The listing builds one solid part. Answer for the finished solid, in the listing's coordinates (mm). A direction names the side the tool comes from. Coordinates: 2 decimals unless noted, no trailing zeros. Loops run counter-clockwise (first coordinate to the right, second up) from the corner with the lowest first, then second, coordinate; pieces in that order, holes last. Notation, with made-up numbers: (51.5, 83) -> (86.5, 83) arc R20 ccw to (86.5, 95) -> close; hole circle Ø11 at (79.5, 50). An arc over 180 degrees is marked (long way). Answer in a Markdown table with one row per item.
Autodesk Inventor part; units mm, degrees
ref_plane "YZ Plane" through (0, 0, 0) normal (1, 0, 0) x (0, 1, 0)
ref_plane "XZ Plane" through (0, 0, 0) normal (0, 1, 0) x (-1, 0, 0)
ref_plane "XY Plane" through (0, 0, 0) normal (0, 0, 1) x (1, 0, 0)
sketch "Sketch1" plane through (0, 0, 0) normal (1, 0, 0) x (0, 1, 0)
  line L0 (0, 0) -> (21.5, 0)
  line L1 (21.5, 0) -> (21.5, -6.35) construction
  line L2 (21.5, -27.85) -> (0, -27.85)
  line L3 (0, -27.85) -> (0, -6.35) construction
  line L4 (21.5, 0) -> (27.85, 0)
  line L5 (27.85, 0) -> (27.85, -34.2)
  line L6 (-6.35, -34.2) -> (-6.35, -6.35) construction
  line L7 (-6.35, 0) -> (0, 0)
  line L8 (27.85, -34.2) -> (-6.35, -34.2)
  line L9 (-6.35, 0) -> (-57.15, 0)
  line L10 (-57.15, 0) -> (-57.15, -82.55)
  line L11 (-6.35, -6.35) -> (-50.8, -6.35)
  line L12 (-50.8, -6.35) -> (-50.8, -76.2)
  line L13 (-6.35, -6.35) -> (-6.35, 0) construction
  line L14 (-57.15, -82.55) -> (-3.7197, -82.55)
  line L15 (-50.8, -76.2) -> (-6.35, -76.2)
  line L16 (-6.35, -76.2) -> (11.6105, -58.2395)
  line L17 (-3.7197, -82.55) -> (11.6105, -67.2197)
  line L18 (11.6105, -58.2395) -> (11.6105, -67.2197)
  line L19 (-6.35, -34.2) -> (-6.35, -76.2) construction
  line L20 (0, -6.35) -> (21.5, -6.35)
  line L21 (0, -6.35) -> (-6.35, -6.35)
  line L22 (0, -6.35) -> (0, 0) construction
  line L23 (21.5, -6.35) -> (21.5, -27.85)
  line L24 (0, -27.85) -> (-6.35, -34.2)
  dimension "d2" = 6.35
  dimension "d4" = 6.35
  dimension "d23" = 6.35
  dimension "d24" = 50.8
  dimension "d25" = 82.55
  dimension "d26" = 6.35
  dimension "d27" = 6.35
  dimension "d28" = 6.35
  dimension "d30" = 6.35
  dimension "d31" = 25.4
  dimension "d32" = 135
  dimension "d33" = 21.5
  dimension "d34" = 6.35
  dimension "d35" = 21.5
  dimension "d36" = 24.0395
extrude "Extrusion1" add sketch "Sketch1" along normal blind 6.35
equation "\"d35\" = d33"
properties part number "Main"
Item 1: A cutting plane is placed at B-B, the plane y = -31.5. Determine the outline of the cut face in (x, z).
Findings below:
| item | result |
|---|---|
| outline | (0, -82.55) -> (6.35, -82.55) -> (6.35, -76.2) -> (0, -76.2) -> close; (0, -6.35) -> (6.35, -6.35) -> (6.35, 0) -> (0, 0) -> close |
Item 2: A cutting plane is placed at D-D, the plane y = -2.5. Determine the outline of the cut face in (x, z).
Findings below:
| item | result |
|---|---|
| outline | (0, -81.33) -> (6.35, -81.33) -> (6.35, -72.35) -> (0, -72.35) -> close; (0, -34.2) -> (6.35, -34.2) -> (6.35, -30.35) -> (0, -30.35) -> close; (0, -6.35) -> (6.35, -6.35) -> (6.35, 0) -> (0, 0) -> close |
Item 3: Find the intervals of material crossed by probe 1 along Y at (x, z) = (5.25, -18.5); probe 2 along Z at (x, y) = (4.5, -18); probe 3 along Z at (x, y) = (4, 6), in increasing order.
Findings below:
| item | result |
|---|---|
| probe 1 | y = -57.15 to -50.8, 21.5 to 27.85 |
| probe 2 | z = -82.55 to -76.2, -6.35 to 0 |
| probe 3 | z = -72.83 to -63.85, -34.2 to -27.85, -6.35 to 0 |
Item 4: Determine the mould class of faces 4 (the face through (0, 1, -29)), 5 (the face through (3.13, 2.5, -67.35)), 6 (the face through (3, -14, 0)) for opening direction Z: +Z half, -Z half, draft (parallel to the pull), parting line (faces both ways), or undercut.
Findings below:
| item | result |
|---|---|
| face 4 | draft |
| face 5 | undercut |
| face 6 | +Z half |
Item 5: A tool of negligible diameter and unlimited length cuts with its end or side. For faces 1 (the face through (3, 11, -34.2)), 2 (the face through (3, 21.5, -17)), 3 (the face through (3, 11.61, -63)), from which of +Z, -Z, +X, -X, +Y, -Y can it reach the whole face along a straight path? Write none if from no direction.
Findings below:
| item | result |
|---|---|
| face 1 | +X, -X, +Y |
| face 2 | +X, -X |
| face 3 | -Z, +X, -X, +Y |
Item 6: A cutting plane is placed at C-C, the plane x = 2.25. Determine the outline of the cut face in (y, z), plus the area to 3 significant figures.
Findings below:
| item | result |
|---|---|
| outline | (-57.15, -82.55) -> (-3.72, -82.55) -> (11.61, -67.22) -> (11.61, -58.24) -> (-6.35, -76.2) -> (-50.8, -76.2) -> (-50.8, -6.35) -> (21.5, -6.35) -> (21.5, -27.85) -> (0, -27.85) -> (-6.35, -34.2) -> (27.85, -34.2) -> (27.85, 0) -> (-57.15, 0) -> close |
| area | 1,800 mm2 |
Item 7: Flat-ended cylindrical pins translate along their axes: pin 1 Ø3 at (x, z) = (3.5, -37) entering from +Y; pin 2 Ø1.5 at (x, y) = (1.5, -13) entering from +Z; pin 3 Ø6 at (y, z) = (-8, -71.5) entering from -X. Find the tip coordinate at first contact, or state that the pin passes through.
Findings below:
| item | result |
|---|---|
| pin 1 | stops at y = -50.8 |
| pin 2 | stops at z = 0 |
| pin 3 | passes through |
Item 8: A cutting plane is placed at A-A, the plane z = -59.5. Determine the outline of the cut face in (x, y).
Findings below:
| item | result |
|---|---|
| outline | (0, -57.15) -> (6.35, -57.15) -> (6.35, -50.8) -> (0, -50.8) -> close; (0, 10.35) -> (6.35, 10.35) -> (6.35, 11.61) -> (0, 11.61) -> close |
